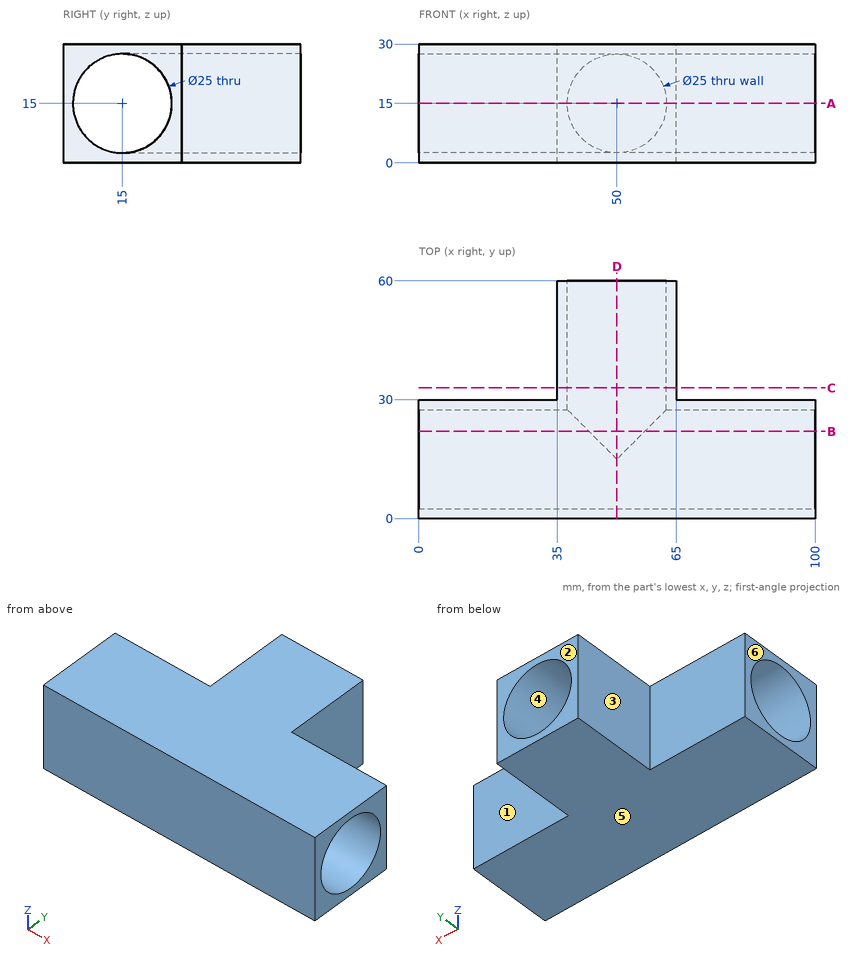
Can you work these out from the drawing? Everything is in mm from the part's minimum corner. A direction names the side the tool comes from. Round coordinates to 2 decimals unless told otherwise and drop trailing zeros. Order: outer loops, then holes, each group sorted by start corner. A loop starts at its lowest first (then second) coordinate and runs counter-clockwise, first axis right, second up. Notation, with made-up numbers: (-32, -32) -> (-16, -32) arc R16 ccw to (-16, -21) -> close; hole circle Ø2 at (0, 48). An arc over 180 degrees is marked (long way). Use CSV: the item, a comma, the result in double quotes.
1. I'm going to push flat-ended pins straight in: P1, Ø1, axis at x = 77.5, z = 17.5, coming from the +Y side; P2, Ø9, axis at y = 40, z = 16.5, coming from the -X side; P3, Ø8, axis at y = 16, z = 9, coming from the +X side. Where does each tip first touch, or does it pass through?
Recorded:
P1,"stops at y = 30"
P2,"stops at x = 35"
P3,"passes through"
2. I want a section at A-A on z = 15. List the corners of the cut face in (x, y) for me.
Recorded:
outline,"(0, 0) -> (100, 0) -> (100, 2.5) -> (0, 2.5) -> close; (0, 27.5) -> (37.5, 27.5) -> (37.5, 60) -> (35, 60) -> (35, 30) -> (0, 30) -> close; (62.5, 27.5) -> (100, 27.5) -> (100, 30) -> (65, 30) -> (65, 60) -> (62.5, 60) -> close"
3. I want a section at D-D on x = 50. List the corners of the cut face in (y, z) for me, and give its area (3 significant figures).
Recorded:
outline,"(0, 0) -> (60, 0) -> (60, 2.5) -> (15, 2.5) arc R12.5 cw to (15, 27.5) -> (60, 27.5) -> (60, 30) -> (0, 30) -> close"
area,"430 mm2"
4. Thinking about a two-plate mould opening in Z: for the marked faces 4, 5 and 6, which applies, pulls with the +Z half, pulls with the -Z half, needs draft (parallel to the pull), parting line crosses it, or undercut?
Recorded:
face 4,"undercut"
face 5,"pulls with the -Z half"
face 6,"needs draft"
5. I want a section at C-C on y = 33. List the corners of the cut face in (x, z) for me.
Recorded:
outline,"(35, 0) -> (65, 0) -> (65, 30) -> (35, 30) -> close; hole circle Ø25 at (50, 15)"
6. I need wall thicknesses on line 1 along Y through (x, z) = (23, 15); line 2 along X through (y, z) = (35, 14.75). Which ranges of each line are inside material? Lowest first, please.
Recorded:
line 1,"y = 0 to 2.5, 27.5 to 30"
line 2,"x = 35 to 37.5, 62.5 to 65"
7. I want a section at B-B on y = 22. List the corners of the cut face in (x, z) for me, and give its area (3 significant figures).
Recorded:
outline,"(0, 0) -> (100, 0) -> (100, 4.64) -> (57, 4.64) arc R12.5 cw to (43, 4.64) -> (0, 4.64) -> close; (0, 25.36) -> (43, 25.36) arc R12.5 cw to (57, 25.36) -> (100, 25.36) -> (100, 30) -> (0, 30) -> close"
area,"888 mm2"
8. Which directions (+Z, -Z, +X, -X, +Y, -Y) give clear straight access to the entire face, cutting with the end or side of a thin tool? Please do the marked faces 1, 2 and 3.
Recorded:
face 1,"+Z, -Z, +X, +Y"
face 2,"+Z, -Z, +X, -X, +Y"
face 3,"+Z, -Z, -X, +Y"
